Part model, mm, in its own coordinate system. A direction names the side the tool comes from. Coordinates: 2 decimals unless noted, no trailing zeros. Order: outer loops, then holes, each group sorted by start corner. A loop starts at its lowest first (then second) coordinate and runs counter-clockwise, first axis right, second up.
from build123d import *

# Parameters (mm, degrees)
BOSS_EXTRUDE1_DEPTH = 80
SKETCH2_R           = 5.0115
CUT_EXTRUDE1_DEPTH  = 80
CUT_EXTRUDE2_DEPTH  = 80


with BuildPart() as part:
    # Sketch1 → Boss-Extrude1 (new body)
    with BuildSketch(Plane.XY):
        Polygon((-42.913522538, 50.7), (-42.913522538, -29.3), (7.086477462, -29.3), (7.086477462, -25.3), (-38.913522538, -25.3), (-38.913522538, 50.7), align=None)
    extrude(amount=BOSS_EXTRUDE1_DEPTH)

    # Sketch2 → Cut-Extrude1 (cut)
    with BuildSketch(Plane(origin=(-38.913522538, 0, 0), x_dir=(0, 0, -1), z_dir=(1, 0, 0))):
        with Locations(Location((-40, 12.7, 0), (0, 0, 90))):
            Circle(SKETCH2_R)
    extrude(amount=-CUT_EXTRUDE1_DEPTH, mode=Mode.SUBTRACT)

    # Sketch3 → Cut-Extrude2 (cut)
    with BuildSketch(Plane(origin=(0, 0, 0), x_dir=(0, 0, -1), z_dir=(1, 0, 0))):
        Polygon((-80, -4.267166785), (-52.498027081, 50.7), (-80, 50.7), align=None)
        Polygon((0, -4.267166785), (-22.400737376, 50.7), (0, 50.7), align=None)
    extrude(amount=-CUT_EXTRUDE2_DEPTH, mode=Mode.SUBTRACT)


solid = part.part
Q1. Cut at D-D on z = 27. Write the cut outline in (x, y).
Results list:
outline: (-42.91, -29.3) - (7.09, -29.3) - (7.09, -25.3) - (-38.91, -25.3) - (-38.91, 50.7) - (-42.91, 50.7) - close
Q2. Which spindle directions (+Z, -Z, +X, -X, +Y, -Y) get a long thin tool onto all of the face, cutting with end or side? Do faces 1 (the face through (-40.886, 22.832, 11.044)), 2 (the face through (-16, -25.3, 39)). Say none if no direction does.
Results list:
face 1: -Z, +X, -X, +Y
face 2: +Z, -Z, +X, +Y
Q3. Wall check: line 1 along Y through (x, z) = (-29, 21.5); line 2 along X through (y, z) = (29.5, 28.5); line 3 along Z through (x, y) = (-40, 12). Give the ranges that are in metal, low to high.
Results list:
line 1: y = -29.3 to -25.3
line 2: x = -42.91 to -38.91
line 3: z = 6.63 to 35.04, 44.96 to 71.86
Q4. Cut at B-B on y = 12.7. Write the cut outline in (x, z).
Results list:
outline: (-42.91, 6.91) - (-38.91, 6.91) - (-38.91, 34.99) - (-42.91, 34.99) - close; (-42.91, 45.01) - (-38.91, 45.01) - (-38.91, 71.51) - (-42.91, 71.51) - close
Q5. Pin check, flat tips, straight feed: pin 1 Ø2 at (x, z) = (-9.5, 8.5) entering from +Y; pin 2 Ø2 at (y, z) = (21, 9) entering from +X. Stop position of each tip, or through.
Results list:
pin 1: stops at y = -25.3
pin 2: passes through
Q6. Cut at A-A on z = 40. Write the cut outline in (x, y).
Results list:
outline: (-42.91, -29.3) - (7.09, -29.3) - (7.09, -25.3) - (-38.91, -25.3) - (-38.91, 7.69) - (-42.91, 7.69) - close; (-42.91, 17.71) - (-38.91, 17.71) - (-38.91, 50.7) - (-42.91, 50.7) - close
Q7. Cut at C-C on x = -16. Write the cut outline in (y, z), and give its area (3 significant figures).
Results list:
outline: (-29.3, 0) - (-25.3, 0) - (-25.3, 80) - (-29.3, 80) - close
area: 320 mm2
Q8. Mould opens along Y. For faces 3 (the face through (-40.89, 17.48, 41.51)), 4 (the face through (-38.914, 4, 39)), 5 (the face through (-40.886, 22.832, 66.442)) say: pulls with the +Y half, pulls with the -Y half, needs draft (parallel to the pull), parting line crosses it, or undercut.
Results list:
face 3: undercut
face 4: needs draft
face 5: pulls with the +Y half
